Input: part model. Units: mm. Frame: model coordinates. A direction names the side the tool comes from. Give positions to 0.01 mm unless a question says otherwise; leave off trailing zeros. Loops run counter-clockwise (first coordinate to the right, second up) from the corner with the lowest first, then second, coordinate; pieces in that order, holes last. Notation, with made-up numbers: (-10, -9) - (20, -9) arc R29 cw to (20, 12) - close; hole circle Ø9 at (15, 12). An arc over 180 degrees is marked (long way). Answer as a JSON object with one key per item and string values.
from build123d import *

# Parameters (mm, degrees)
F0_R     = 12.7
F1_DEPTH = 127
F5_DEPTH = 25.4


# Not quite as in the source:
# - the program builds the solid bodies; features that only make, move or delete a surface that nothing else refers to are left out


with BuildPart() as f1:
    # F0 (on Front) → F1 (new body)
    with BuildSketch(Plane.XZ):
        with Locations((48.1354147196, 27.8021357954)):
            Circle(F0_R)
    extrude(amount=F1_DEPTH)

    # F2 (on face) → F5 (join)
    with BuildSketch(Plane(origin=(0, 0, 0), x_dir=(-1, 0, 0), z_dir=(0, 1, 0))):
        with BuildLine():
            Line((-49.2203550876, 40.4557085872), (-60.73924371, 40.4557085872))
            Line((-60.73924371, 40.4557085872), (-60.73924371, 29.3621020704))
            ThreePointArc((-60.73924371, 29.3621020704), (-56.94521767, 36.9496694507), (-49.2203550876, 40.4557085872))
        make_face()
        with BuildLine():
            Line((-35.33924371, 40.4557085872), (-47.0504743515, 40.4557085872))
            ThreePointArc((-47.0504743515, 40.4557085872), (-38.7794342078, 36.3902455212), (-35.4354147196, 27.8021357954))
            ThreePointArc((-35.4354147196, 27.8021357954), (-47.3539507661, 15.126201349), (-60.73924371, 26.2421695203))
            Line((-60.73924371, 26.2421695203), (-60.73924371, 15.0557085872))
            Line((-60.73924371, 15.0557085872), (-35.33924371, 15.0557085872))
            Line((-35.33924371, 15.0557085872), (-35.33924371, 40.4557085872))
        make_face()
        with BuildLine():
            Line((-47.0504743515, 40.4557085872), (-49.2203550876, 40.4557085872))
            ThreePointArc((-49.2203550876, 40.4557085872), (-56.94521767, 36.9496694507), (-60.73924371, 29.3621020704))
            Line((-60.73924371, 29.3621020704), (-60.73924371, 26.2421695203))
            ThreePointArc((-60.73924371, 26.2421695203), (-47.3539507661, 15.126201349), (-35.4354147196, 27.8021357954))
            ThreePointArc((-35.4354147196, 27.8021357954), (-38.7794342078, 36.3902455212), (-47.0504743515, 40.4557085872))
        make_face()
    extrude(amount=F5_DEPTH)


solid = f1.part
Item 1: Contact query for flat-ended pins moving along their axis: P1, Ø1, axis at y = -76, z = 30, coming from the -X side; P2, Ø12, axis at y = -108, z = 31.5, coming from the -X side; P3, Ø12.5, axis at y = 6.5, z = 22.5, coming from the +X side. Output: stop coordinate, or through.
Geometry check:
{"P1": "stops at x = 35.55", "P2": "stops at x = 35.44", "P3": "stops at x = 60.74"}
Item 2: Cut plane C-C (y = -41). Return loops of the section in (x, z), then the cut area to 3 significant figures.
Geometry check:
{"outline": "circle Ø25.4 at (48.14, 27.8)", "area": "507 mm2"}
Item 3: Access query for faces 1 (the face through (58, 0, 38)), 2 (the face through (41, 0, 17)), 3 (the face through (48, 13, 15.056)). Directions: +Z, -Z, +X, -X, +Y, -Y. A direction counts if a zero-diameter tool reaches every point of the face in a straight line with its end or side. Return the directions, or none.
Geometry check:
{"face 1": "+Z, +X, -Y", "face 2": "-Y", "face 3": "-Z, +X, -X, +Y, -Y"}
Item 4: Material intervals for line 1 (Z direction, x = 47.5, y = 1); line 2 (X direction, y = -71.5, z = 28.5); line 3 (X direction, y = 7, z = 38.75), sorted ascending. Write a range as [from, to].
Geometry check:
{"line 1": "z = [15.06, 40.46]", "line 2": "x = [35.45, 60.82]", "line 3": "x = [35.34, 60.74]"}
Item 5: Cut plane B-B (z = 31.5). Return loops of the section in (x, y).
Geometry check:
{"outline": "(35.34, 0) - (35.99, 0) - (35.99, -127) - (60.29, -127) - (60.29, 0) - (60.74, 0) - (60.74, 25.4) - (35.34, 25.4) - close"}
Item 6: Cut plane A-A (x = 45.5). Return loops of the section in (y, z), then the cut area to 3 significant figures.
Geometry check:
{"outline": "(-127, 15.38) - (0, 15.38) - (0, 15.06) - (25.4, 15.06) - (25.4, 40.46) - (0, 40.46) - (0, 40.23) - (-127, 40.23) - close", "area": "3,800 mm2"}
